Check sheet for the modelled part. Datum: model origin and axes. Units: mm. A direction names the side the tool comes from. Round coordinates to 2 decimals unless told otherwise and drop trailing zeros. Order: outer loops, then holes, each group sorted by start corner. A loop starts at its lowest first (then second) coordinate and runs counter-clockwise, first axis right, second up.
```python
from build123d import *

# Parameters (mm, degrees)
F1_DEPTH = 3
F0_W     = 39.9216501117
F0_H     = 3
F0_W_2   = 3
F0_H_2   = 40
F0_W_3   = 40
F0_H_3   = 40.3722185198
F2_DEPTH = 4
F0_W_4   = 7
F0_H_4   = 9
F0_W_5   = 9
F0_H_5   = 7
F3_DEPTH = 2
F4_DEPTH = 8
F0_H_6   = 4
F0_W_6   = 4
F5_DEPTH = 11
F6_SIZE  = 4.99999


# Not quite as in the source:
# - a fillet or chamfer is up to 0.001 mm smaller than in the source, because OpenCascade refuses the exact size


with BuildPart() as f1:
    # F0 (on Top) → F1 (new body)
    with BuildSketch(Plane.XY):
        Polygon((-71.7994198203, 65.224928081), (-71.7994198203, 68.224928081), (-84, 68.224928081), (-84, -2.7506086044), (-77, -2.7506086044), (-77, -19.5105448365), (-84, -19.5105448365), (-84, -30.4028533991), (-81, -30.4028533991), (-81, -34.4028533991), (-88, -34.4028533991), (-88, -74.775071919), (-81, -74.775071919), (-81, -78.775071919), (-84, -78.775071919), (-84, -90.775071919), (-12, -90.775071919), (-12, -83.775071919), (3, -83.775071919), (3, -90.775071919), (15, -90.775071919), (15, -87.775071919), (19, -87.775071919), (19, -94.775071919), (59, -94.775071919), (59, -87.775071919), (63, -87.775071919), (63, -90.775071919), (75, -90.775071919), (75, -18.775071919), (68.6397999525, -18.775071919), (68, -18.775071919), (68, -3.775071919), (75, -3.775071919), (75, 8.224928081), (69.781611979, 8.224928081), (69.781611979, 12.224928081), (77.218388021, 12.224928081), (77.218388021, 52.224928081), (69.781611979, 52.224928081), (70.218388021, 56.224928081), (75, 56.224928081), (75, 68.224928081), (3.8335430436, 68.224928081), (3.8335430436, 61.224928081), (-12.6577513292, 61.224928081), (-12.6577513292, 68.224928081), (-23.8777697086, 68.224928081), (-23.8777697086, 65.224928081), (-27.8777697086, 65.224928081), (-27.8777697086, 72.224928081), (-67.7994198203, 72.224928081), (-67.7994198203, 65.224928081), align=None)
    extrude(amount=F1_DEPTH)

    # F0 (on Top) → F2 (join)
    with BuildSketch(Plane.XY):
        Polygon((-74.8768895864, 71.224928081), (-87, 71.224928081), (-87, 59.224928081), (-91, 59.224928081), (-91, 56.224928081), (-87, 56.224928081), (-87, 51.624928081), (-91, 51.624928081), (-91, 12.824928081), (-87, 12.824928081), (-87, 8.224928081), (-91, 8.224928081), (-91, 5.224928081), (-87, 5.224928081), (-87, -6.775071919), (-80, -6.775071919), (-80, -15.775071919), (-87, -15.775071919), (-87, -27.4028533991), (-91, -27.4028533991), (-91, -30.4028533991), (-84, -30.4028533991), (-84, -19.5105448365), (-77, -19.5105448365), (-77, -2.7506086044), (-84, -2.7506086044), (-84, 68.224928081), (-71.7994198203, 68.224928081), (-71.7994198203, 75.224928081), (-74.8768895864, 75.224928081), align=None)
        with Locations((-47.8385947645, 73.724928081)):
            Rectangle(F0_W, F0_H)
        Polygon((-20.8768895864, 75.224928081), (-23.8777697086, 75.224928081), (-23.8777697086, 68.224928081), (-12.6577513292, 68.224928081), (-12.6577513292, 61.224928081), (3.8335430436, 61.224928081), (3.8335430436, 68.224928081), (75, 68.224928081), (75, 56.224928081), (80.218388021, 56.224928081), (80.218388021, 59.224928081), (78, 59.224928081), (78, 71.224928081), (66, 71.224928081), (66, 75.224928081), (62.9867989421, 75.224928081), (63, 71.224928081), (58.4, 71.224928081), (58.3867989421, 75.224928081), (19.6, 75.224928081), (19.6, 71.224928081), (15, 71.224928081), (15, 75.224928081), (12, 75.224928081), (12, 71.224928081), (0, 71.224928081), (0, 64.224928081), (-9, 64.224928081), (-9, 71.224928081), (-20.8768895864, 71.224928081), align=None)
        with Locations((78.718388021, 32.224928081)):
            Rectangle(F0_W_2, F0_H_2)
        Polygon((79.781611979, 8.224928081), (75, 8.224928081), (75, -3.775071919), (68, -3.775071919), (68, -18.775071919), (68.6397999525, -18.775071919), (75, -18.775071919), (75, -90.775071919), (63, -90.775071919), (63, -97.775071919), (66, -97.775071919), (66, -93.775071919), (78, -93.775071919), (78, -81.775071919), (83.6185051799, -81.775071919), (83.6185051799, -78.775071919), (78, -78.775071919), (78, -74.175071919), (83.6185051799, -74.175071919), (83.6185051799, -35.375071919), (78, -35.375071919), (78, -30.775071919), (83.6185051799, -30.775071919), (83.6185051799, -27.775071919), (78, -27.775071919), (78, -15.775071919), (71, -15.775071919), (71, -6.775071919), (78, -6.775071919), (78, 5.224928081), (80.218388021, 5.224928081), (80.218388021, 8.224928081), align=None)
        with Locations((39, -96.275071919)):
            Rectangle(F0_W_3, F0_H)
        Polygon((-84, -90.775071919), (-84, -78.775071919), (-91, -78.775071919), (-91, -81.775071919), (-87, -81.775071919), (-87, -93.775071919), (-75, -93.775071919), (-75, -97.775071919), (-72, -97.775071919), (-72, -93.775071919), (-67.4, -93.775071919), (-67.4, -97.775071919), (-28.6, -97.775071919), (-28.6, -93.775071919), (-24, -93.775071919), (-24, -97.775071919), (-21, -97.775071919), (-21, -93.775071919), (-9, -93.775071919), (-9, -86.775071919), (0, -86.775071919), (0, -93.775071919), (12, -93.775071919), (12, -97.775071919), (15, -97.775071919), (15, -97.4028533991), (15, -90.775071919), (3, -90.775071919), (3, -83.775071919), (-12, -83.775071919), (-12, -90.775071919), align=None)
        with Locations((-89.5, -54.5889626591)):
            Rectangle(F0_W_2, F0_H_3)
    extrude(amount=F2_DEPTH)

    # F0 (on Top) → F3 (join)
    with BuildSketch(Plane.XY):
        with Locations((-83.5, -11.275071919)):
            Rectangle(F0_W_4, F0_H_4)
        with Locations((-4.5, 67.724928081)):
            Rectangle(F0_W_5, F0_H_5)
        with Locations((74.5, -11.275071919)):
            Rectangle(F0_W_4, F0_H_4)
        with Locations((-4.5, -90.275071919)):
            Rectangle(F0_W_5, F0_H_5)
    extrude(amount=F3_DEPTH)

    # F0 (on Top) → F4 (join)
    with BuildSketch(Plane.XY):
        Polygon((-71.7994198203, 78.224928081), (-71.7994198203, 75.224928081), (-71.7994198203, 68.224928081), (-71.7994198203, 65.224928081), (-67.7994198203, 65.224928081), (-67.7994198203, 72.224928081), (-67.7994198203, 75.224928081), (-67.7994198203, 78.224928081), align=None)
        Polygon((-27.8777697086, 78.224928081), (-27.8777697086, 75.224928081), (-27.8777697086, 72.224928081), (-27.8777697086, 65.224928081), (-23.8777697086, 65.224928081), (-23.8777697086, 68.224928081), (-23.8777697086, 75.224928081), (-23.8777697086, 78.224928081), align=None)
        Polygon((80.218388021, 56.224928081), (75, 56.224928081), (70.218388021, 56.224928081), (69.781611979, 52.224928081), (77.218388021, 52.224928081), (80.218388021, 52.224928081), (83.218388021, 52.224928081), (83.218388021, 56.224928081), align=None)
        Polygon((80.218388021, 12.224928081), (77.218388021, 12.224928081), (69.781611979, 12.224928081), (69.781611979, 8.224928081), (75, 8.224928081), (79.781611979, 8.224928081), (80.218388021, 8.224928081), (83.218388021, 8.224928081), (83.218388021, 12.224928081), align=None)
        Polygon((59, -87.775071919), (59, -94.775071919), (59, -97.775071919), (59, -100.775071919), (63, -100.775071919), (63, -97.775071919), (63, -90.775071919), (63, -87.775071919), align=None)
        Polygon((15, -87.775071919), (15, -90.775071919), (15, -97.4028533991), (15, -97.775071919), (15, -100.775071919), (19, -100.775071919), (19, -97.775071919), (19, -94.775071919), (19, -87.775071919), align=None)
        Polygon((-81, -30.4028533991), (-84, -30.4028533991), (-91, -30.4028533991), (-94, -30.4028533991), (-94, -34.4028533991), (-91, -34.4028533991), (-88, -34.4028533991), (-81, -34.4028533991), align=None)
        Polygon((-81, -74.775071919), (-88, -74.775071919), (-91, -74.775071919), (-91.2415088892, -74.775071919), (-94, -74.775071919), (-94, -78.775071919), (-91, -78.775071919), (-84, -78.775071919), (-81, -78.775071919), align=None)
    extrude(amount=F4_DEPTH)

    # F0 (on Top) → F5 (join)
    with BuildSketch(Plane.XY):
        with Locations((-95.5, -32.4028533991)):
            Rectangle(F0_W_2, F0_H_6)
        with Locations((-95.5, -76.775071919)):
            Rectangle(F0_W_2, F0_H_6)
        with Locations((17, -102.275071919)):
            Rectangle(F0_W_6, F0_H)
        with Locations((61, -102.275071919)):
            Rectangle(F0_W_6, F0_H)
        with Locations((84.718388021, 10.224928081)):
            Rectangle(F0_W_2, F0_H_6)
        with Locations((84.718388021, 54.224928081)):
            Rectangle(F0_W_2, F0_H_6)
        with Locations((-25.8777697086, 79.724928081)):
            Rectangle(F0_W_6, F0_H)
        with Locations((-69.7994198203, 79.724928081)):
            Rectangle(F0_W_6, F0_H)
    extrude(amount=F5_DEPTH)

    # F6 (size 5 in the source; OpenCascade refuses exactly that, so slightly less here)
    f6_edges = [f1.edges().sort_by_distance(p)[0] for p in [
        (-69.79942, 65.224928, 8),
        (-25.87777, 65.224928, 8),
        (70, 54.224928, 8),
        (69.781612, 10.224928, 8),
        (-81, -76.775072, 8),
        (-81, -32.402853, 8),
        (61, -87.775072, 8),
        (17, -87.775072, 8),
    ]]
    chamfer(f6_edges, length=F6_SIZE)


solid = f1.part
```
Item 1: Sectioned sample at A-A (x = 26). Record the cut outline in (y, z).
Answer:
outline: (-97.78, 0) - (75.22, 0) - (75.22, 4) - (68.22, 4) - (68.22, 3) - (-94.78, 3) - (-94.78, 4) - (-97.78, 4) - close
Item 2: Go/stop test with flat-tipped pins: P1, Ø3, axis at y = -61, z = 3, coming from the -X side; P2, Ø1.1, axis at y = -8.5, z = 3.5, coming from the +X side; P3, Ø1.2, axis at x = 79.5, z = 2, coming from the -Y side; P4, Ø10, axis at x = -66, y = -53, coming from the -Z side. Record where each tip stops, or that it passes through.
Answer:
P1: stops at x = -91
P2: stops at x = 71
P3: stops at y = -81.78
P4: stops at z = 0
Item 3: Scan lines: line 1 along X through (y, z) = (72, 6.5); line 2 along Z through (x, y) = (-34, 55.5); line 3 along X through (y, z) = (-22, 3.5). Record each from-to range of solid material in increasing order.
Answer:
line 1: x = -71.8 to -67.8, -27.88 to -23.88
line 2: z = 0 to 3
line 3: x = -87 to -84, 75 to 78
Item 4: Release check for a two-part mould opening along Y. For faces 6 (the flat face through (-48, 75.225, 2)), 7 (the flat face through (-91, 32, 2)), 8 (the flat face through (-89, 5.225, 2)), 9 (the flat face through (82, 12.225, 5)) record: released by +Y, released by -Y, zero draft, split by the parting line, or undercut.
Answer:
face 6: released by +Y
face 7: zero draft
face 8: undercut
face 9: undercut
Item 5: Sectioned sample at C-C (x = -6). Record the cut outline in (y, z), and give its area (3 significant figures).
Answer:
outline: (-93.78, 0) - (71.22, 0) - (71.22, 2) - (64.22, 2) - (64.22, 4) - (61.22, 4) - (61.22, 3) - (-83.78, 3) - (-83.78, 4) - (-86.78, 4) - (-86.78, 2) - (-93.78, 2) - close
area: 487 mm2
Item 6: Sectioned sample at B-B (y = -22.5). Record the cut outline in (x, z), and give its area (3 significant figures).
Answer:
outline: (-87, 0) - (78, 0) - (78, 4) - (75, 4) - (75, 3) - (-84, 3) - (-84, 4) - (-87, 4) - close
area: 501 mm2
Item 7: Access from +Z, -Z, +X, -X, +Y, -Y to the whole of each face (thin tool, end or side, straight path). Record for faces 1 (the flat face through (-26, 74, 8)), 2 (the flat face through (-26, -93.775, 2)), 3 (the flat face through (81, -30.775, 2)), 4 (the flat face through (-5, -90, 2)), 5 (the flat face through (19.6, 73, 2)).
Answer:
face 1: +Z, +X, -X, -Y
face 2: +Z, -Z, -Y
face 3: +Z, -Z, +X
face 4: +Z, -Y
face 5: +Z, -Z, +Y
